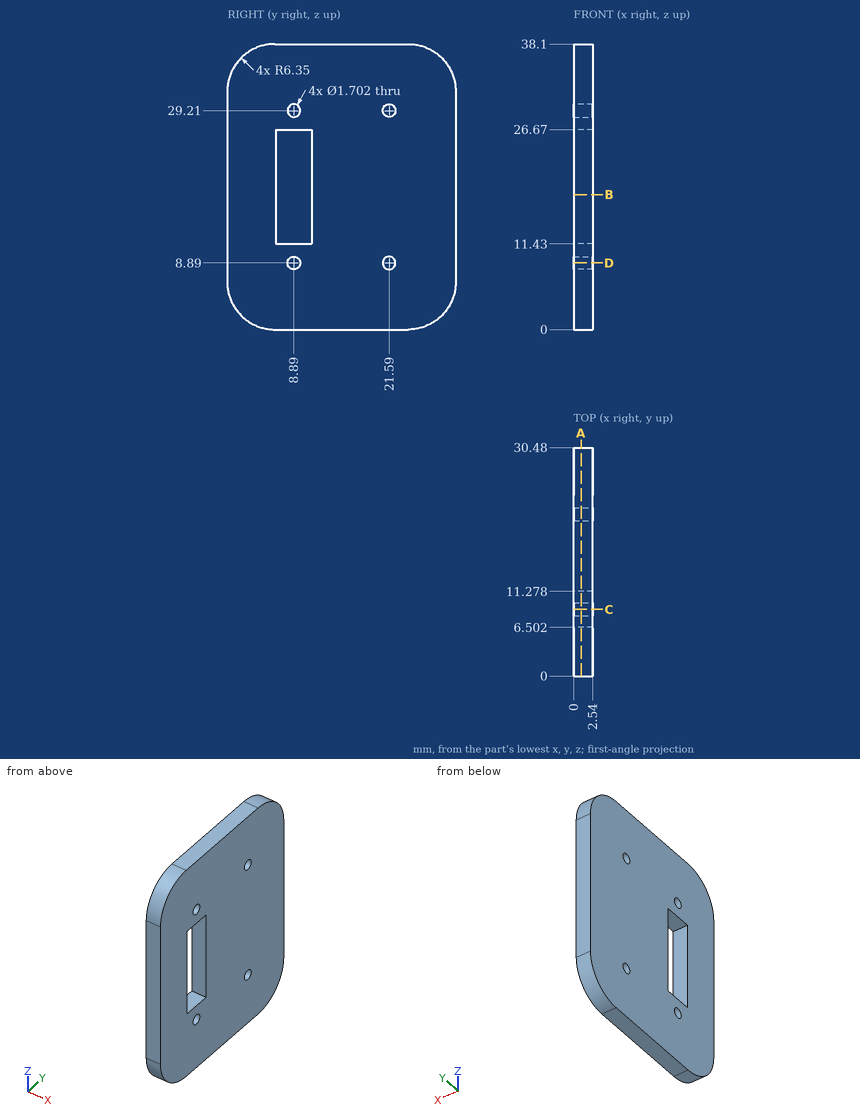
Geometry: see drawing. Coordinates: mm, zero at the bounding-box minimum. Coordinates: 2 decimals unless noted, no trailing zeros. Loops run counter-clockwise (first coordinate to the right, second up) from the corner with the lowest first, then second, coordinate; pieces in that order, holes last. Notation, with made-up numbers: (55, 40.5) - (93, 40.5) arc R22 cw to (93, 72.5) - close; hole circle Ø6 at (26, -19.75). An arc over 180 degrees is marked (long way). Put each result on its own line as item: value. Start each with the question number.
Q1. Cut plane C-C, the plane y = 8.89. Return loops of the section in (x, z).
Q2. Cut plane A-A, the plane x = 1. Return loops of the section in (y, z).
Q3. Cut plane D-D, the plane z = 8.89. Return loops of the section in (x, y).
Q4. Pin query (flat end, axial travel): pin 1 Ø1 at (x, y) = (0.5, 20.5) entering from -Z; pin 2 Ø1.4 at (y, z) = (8.89, 29.21) entering from -X. Return the tip coordinate at first contact, or that it passes through.
Q5. Line query: line 1 (Y direction, x = 0.55, z = 8.89); line 2 (Y direction, x = 2.45, z = 15.5); line 3 (Z direction, x = 1.45, y = 8). Output: solid intervals per line, ascending.
Q6. Cut plane B-B, the plane z = 18. Return loops of the section in (x, y).
Filled sheet:
1. outline: (0, 0) - (2.54, 0) - (2.54, 8.04) - (0, 8.04) - close; (0, 9.74) - (2.54, 9.74) - (2.54, 11.43) - (0, 11.43) - close; (0, 26.67) - (2.54, 26.67) - (2.54, 28.36) - (0, 28.36) - close; (0, 30.06) - (2.54, 30.06) - (2.54, 38.1) - (0, 38.1) - close
2. outline: (0, 6.35) arc R6.35 ccw to (6.35, 0) - (24.13, 0) arc R6.35 ccw to (30.48, 6.35) - (30.48, 31.75) arc R6.35 ccw to (24.13, 38.1) - (6.35, 38.1) arc R6.35 ccw to (0, 31.75) - close; hole (6.5, 11.43) - (11.28, 11.43) - (11.28, 26.67) - (6.5, 26.67) - close; hole circle Ø1.7 at (8.89, 8.89); hole circle Ø1.7 at (8.89, 29.21); hole circle Ø1.7 at (21.59, 8.89); hole circle Ø1.7 at (21.59, 29.21)
3. outline: (0, 0) - (2.54, 0) - (2.54, 8.04) - (0, 8.04) - close; (0, 9.74) - (2.54, 9.74) - (2.54, 20.74) - (0, 20.74) - close; (0, 22.44) - (2.54, 22.44) - (2.54, 30.48) - (0, 30.48) - close
4. pin 1: z = 0
4. pin 2: through
5. line 1: 0 to 8.04, 9.74 to 20.74, 22.44 to 30.48
5. line 2: 0 to 6.5, 11.28 to 30.48
5. line 3: 0 to 11.43, 26.67 to 38.1
6. outline: (0, 0) - (2.54, 0) - (2.54, 6.5) - (0, 6.5) - close; (0, 11.28) - (2.54, 11.28) - (2.54, 30.48) - (0, 30.48) - close
